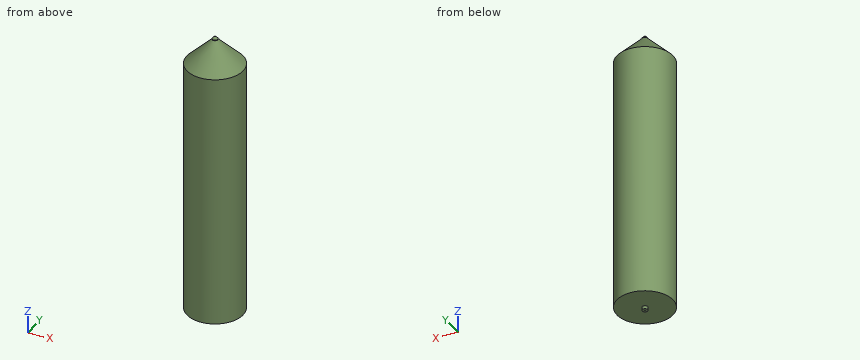
from build123d import *

# Parameters (mm, degrees)
F0_R     = 25.4
F1_DEPTH = 127
F2_SIZE  = 22.86
F4_DEPTH = 254.001
F5_R     = 2.54
F5_R_2   = 0.3020400554
F6_DEPTH = 129.794


# Not quite as in the source:
# - a fillet or chamfer that OpenCascade refuses, or shapes differently, is made with other operations: its cross-section is extruded or revolved along the edge and cut away or added


with BuildPart() as f1:
    # F0 (on Top) → F1 (new body, symmetric)
    with BuildSketch(Plane.XY):
        Circle(F0_R)
    extrude(amount=F1_DEPTH, both=True)

    # F2
    f2_edges = [f1.edges().sort_by_distance(p)[0] for p in [
        (-25.4, 0, 127),
    ]]
    chamfer(f2_edges, length=F2_SIZE)

    # F4 (cut, through all): a face of the model
    f4_faces = [f1.faces().sort_by_distance(p)[0] for p in [
        (0, 0, 127),
    ]]
    extrude(f4_faces, amount=-F4_DEPTH, mode=Mode.SUBTRACT)

    # F5 (on Top) → F6 (join, symmetric)
    with BuildSketch(Plane.XY):
        Circle(F5_R)
        Circle(F5_R_2, mode=Mode.SUBTRACT)
    extrude(amount=F6_DEPTH, both=True)

    # F7: chamfer of 2.286 on 1 edges, made by hand

    # F7_s1 → F7_t2 (revolve, cut)
    with BuildSketch(Plane.XZ):
        Polygon((0.254, 129.794), (2.54, 127.508), (2.54, 129.794), align=None)
    revolve(axis=Axis((0, 0, 129.794), (0, 0, 1)), mode=Mode.SUBTRACT)


solid = f1.part
The listing builds one solid part. Answer for the finished solid, in the listing's coordinates (mm). Give positions to 0.01 mm unless a question says otherwise; leave off trailing zeros. Write each loop counter-clockwise with the first axis right and the second up, starting at its lowest first coordinate (ties: lowest second). Pieces come first, ordered by that corner, then holes. Notation, with made-up numbers: (54.25, -6) - (87.25, -6) arc R7 cw to (87.25, 4) - close; hole circle Ø2 at (44.5, 8.25). An arc over 180 degrees is marked (long way). Use a Markdown table: item, result.
1. Each of these flat-tipped pins is pushed along its axis until it touches: P1, Ø12, axis at x = 3, z = 65, coming from the -Y side; P2, Ø4, axis at x = -1, z = -57.5, coming from the +Y side; P3, Ø2, axis at y = 12, z = -72, coming from the -X side. Where does it stop, or does it pass through?
Values follow:
| item | result |
|---|---|
| P1 | stops at y = -25.4 |
| P2 | stops at y = 25.4 |
| P3 | stops at x = -22.89 |
2. Section A-A on z = 50 is taken. Write down the section's boundary in (x, y).
Values follow:
| item | result |
|---|---|
| outline | circle Ø50.8 at (0, 0); hole circle Ø0.6 at (0, 0) |
3. Find the intervals of material crossed by probe 1 along Y at (x, z) = (0, -11); probe 2 along X at (y, z) = (15, -113.5); probe 3 along X at (y, z) = (-12.5, -104), in increasing order. Write a range as from..to.
Values follow:
| item | result |
|---|---|
| probe 1 | y = -25.4..-0.3, 0.3..25.4 |
| probe 2 | x = -20.5..20.5 |
| probe 3 | x = -22.11..22.11 |
